Model file for the job. Use its own axes, mm. Face numbers are marked on the shaded views. A direction names the side the tool comes from. Give positions to 0.01 mm unless a question says otherwise; leave off trailing zeros. Loops run counter-clockwise (first coordinate to the right, second up) from the corner with the lowest first, then second, coordinate; pieces in that order, holes last. Notation, with made-up numbers: (-32, 84) - (1, 84) arc R14 ccw to (1, 109) - close; hole circle Ø8 at (41.25, 68). An arc over 180 degrees is marked (long way). Use a Markdown table: item, result.
from build123d import *

# Parameters (mm, degrees)
F0_W     = 63.5
F0_H     = 30.5136416812
F0_R     = 1.524
F0_W_2   = 41.529
F0_H_2   = 6.7564
F1_DEPTH = 5.08
F2_W     = 63.5
F2_H     = 8.9645285864
F3_DEPTH = 25.4
F4_W     = 63.5
F4_H     = 8.5140008438
F5_DEPTH = 12.7
F6_R     = 2.3114
F7_DEPTH = 25.4
F8_DEPTH = 21.9659991562


with BuildPart() as f1:
    # F0 (on Top) → F1 (new body)
    with BuildSketch(Plane.XY):
        with Locations((31.75, 15.2568208406)):
            Rectangle(F0_W, F0_H)
        with Locations((2.9337, 14.7922589307)):
            Circle(F0_R, mode=Mode.SUBTRACT)
        with Locations((31.75, 14.7922589307)):
            Rectangle(F0_W_2, F0_H_2, mode=Mode.SUBTRACT)
        with Locations((60.5663, 14.7922589307)):
            Circle(F0_R, mode=Mode.SUBTRACT)
    extrude(amount=F1_DEPTH)

    # F2 (on face) → F3 (join)
    with BuildSketch(Plane.XY.offset(5.08)):
        with Locations((31.75, 26.031377388)):
            Rectangle(F2_W, F2_H)
    extrude(amount=F3_DEPTH)

    # F4 (on face) → F5 (join)
    with BuildSketch(Plane(origin=(0, 30.5136416812, 0), x_dir=(-1, 0, 0), z_dir=(0, 1, 0))):
        with Locations((-31.75, 26.2229995781)):
            Rectangle(F4_W, F4_H)
    extrude(amount=F5_DEPTH)

    # F6 (on face) → F7 (cut)
    with BuildSketch(Plane.XY.offset(30.48)):
        with Locations((57.0266509049, 35.708874464)):
            Circle(F6_R)
        with Locations((6.2266509049, 35.8004383743)):
            Circle(F6_R)
    extrude(amount=-F7_DEPTH, mode=Mode.SUBTRACT)

    # F8 (add, through all): a face of the model
    f8_faces = [f1.faces().sort_by_distance(p)[0] for p in [
        (31.7553573875, 36.9118079348, 21.9659991562),
    ]]
    extrude(f8_faces, amount=F8_DEPTH)


solid = f1.part
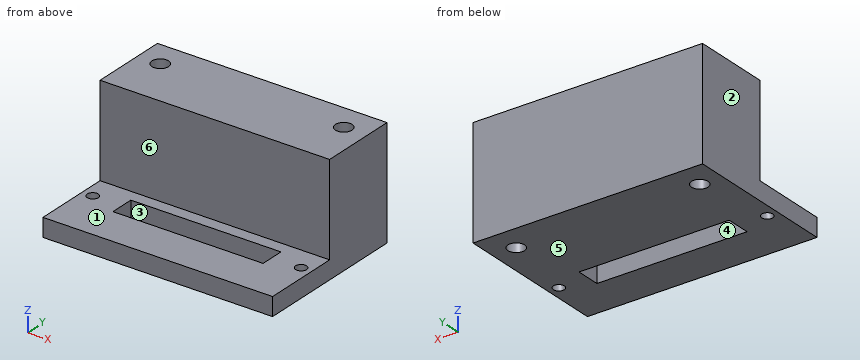
(1) 3-axis set-ups, long thin cutter, end or side, ignore diameter. For the marked faces 4, 5 and 6: which of +Z, -Z, +X, -X, +Y, -Y reach the whole face in a straight line?
Computed:
| item | result |
|---|---|
| face 4 | +Z, -Z |
| face 5 | -Z, +X, -X, +Y, -Y |
| face 6 | +Z, +X, -X, -Y |
(2) Slice it at D-D, the plane y = 8.5. Write the cut outline in (x, z).
Computed:
| item | result |
|---|---|
| outline | (0, 0) - (63.5, 0) - (63.5, 5.08) - (0, 5.08) - close |
(3) Pin check, flat tips, straight feed: P1, Ø3.5, axis at x = 6.23, y = 35.8, coming from the -Z side; P2, Ø11, axis at x = 43.5, y = 8.5, coming from the +Z side; P3, Ø6, axis at x = 44.5, y = 6, coming from the -Z side. Stop position of each tip, or through.
Computed:
| item | result |
|---|---|
| P1 | through |
| P2 | z = 5.08 |
| P3 | z = 0 |
(4) Slice it at A-A, the plane x = 45. Write the cut outline in (y, z), plus the area to 3 significant figures.
Computed:
| item | result |
|---|---|
| outline | (0, 0) - (11.41, 0) - (11.41, 5.08) - (0, 5.08) - close; (18.17, 0) - (43.21, 0) - (43.21, 30.48) - (21.55, 30.48) - (21.55, 5.08) - (18.17, 5.08) - close |
| area | 735 mm² |
(5) Slice it at C-C, the plane x = 58. Write the cut outline in (y, z), plus the area to 3 significant figures.
Computed:
| item | result |
|---|---|
| outline | (0, 0) - (33.61, 0) - (33.61, 30.48) - (21.55, 30.48) - (21.55, 5.08) - (0, 5.08) - close; (37.81, 0) - (43.21, 0) - (43.21, 30.48) - (37.81, 30.48) - close |
| area | 642 mm² |
(6) Drill centre lines: probe 1 along Y at (x, z) = (49, 5); probe 2 along Y at (x, z) = (27, 10.5); probe 3 along Z at (x, y) = (9, 12.5). Where is each one in solid material? Low to high. Write a range as [from, to].
Computed:
| item | result |
|---|---|
| probe 1 | [0, 11.41], [18.17, 43.21] |
| probe 2 | [21.55, 43.21] |
| probe 3 | [0, 5.08] |
(7) Slice it at B-B, the plane z = 4. Write the cut outline in (x, y).
Computed:
| item | result |
|---|---|
| outline | (0, 0) - (63.5, 0) - (63.5, 43.21) - (0, 43.21) - close; hole circle Ø3.05 at (2.93, 14.79); hole circle Ø4.62 at (6.23, 35.8); hole (10.99, 11.41) - (52.51, 11.41) - (52.51, 18.17) - (10.99, 18.17) - close; hole circle Ø4.62 at (57.03, 35.71); hole circle Ø3.05 at (60.57, 14.79) |
(8) Mould opens along X. For the marked faces 1, 2 and 3 say: pulls with the +X half, pulls with the -X half, needs draft (parallel to the pull), parting line crosses it, or undercut.
Computed:
| item | result |
|---|---|
| face 1 | needs draft |
| face 2 | pulls with the -X half |
| face 3 | undercut |
